Geometry check sheet. Reference: drawing and pictorial views, mm from the part's lowest x, y, z. A direction names the side the tool comes from. Round coordinates to 2 decimals unless told otherwise and drop trailing zeros. Write each loop counter-clockwise with the first axis right and the second up, starting at its lowest first coordinate (ties: lowest second). Pieces come first, ordered by that corner, then holes. Notation, with made-up numbers: M 45.5,32.25 L 74.5,32.25 A22 cw 74.5,55.25 Z; hole C 32.25,-14.5 d3. An arc over 180 degrees is marked long. Put each result on its own line as item: value. Start each with the question number.
(1) Section check A-A on x = 57.5. Record the cut outline in (y, z).
(2) Section check C-C on y = 102.5. Record the cut outline in (x, z), then the cut area to 3 significant figures.
(3) Material ranges on probe 1 along Y at (x, z) = (56, 52.5); probe 2 along Y at (x, z) = (57.5, 54); probe 3 along Z at (x, y) = (7.5, 31.5), recorded low to high.
(4) Tool access check on the marked faces 1 and 2. Record the directions out of +Z, -Z, +X, -X, +Y, -Y that give a thin tool (end or side, any length) a straight path to the whole face; none if there is none.
(5) Mould release check, pull along Y, two halves, no side actions. Record for the marked faces 3, 4 and 5: pulls with the +Y half, pulls with the -Y half, needs draft (parallel to the pull), parting line crosses it, or undercut.
(6) Gauge pin test, flat ends, axial feed: pin 1 (6 mm diameter, centred on x = 102.5, y = 57.5, fed in from +Z); pin 2 (10 mm diameter, centred on x = 22.5, z = 46.5, fed in from +Y); pin 3 (10 mm diameter, centred on x = 62.5, z = 6, fed in from -Y); pin 4 (10 mm diameter, centred on x = 65.5, z = 29, fed in from -Y). Record the tip position at first contact, or that the pin passes through.
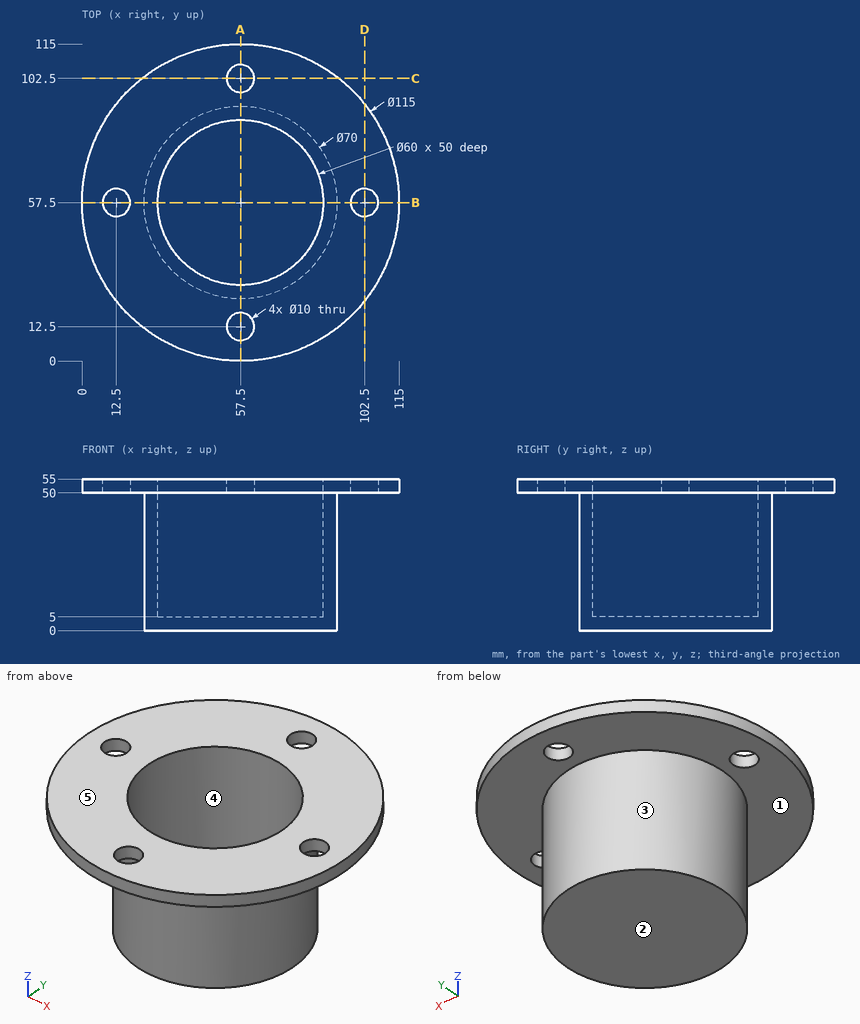
Answers follow:
1. outline: M 0,50 L 7.5,50 L 7.5,55 L 0,55 Z; M 17.5,50 L 22.5,50 L 22.5,0 L 92.5,0 L 92.5,50 L 97.5,50 L 97.5,55 L 87.5,55 L 87.5,5 L 27.5,5 L 27.5,55 L 17.5,55 Z; M 107.5,50 L 115,50 L 115,55 L 107.5,55 Z
2. outline: M 21.71,50 L 52.5,50 L 52.5,55 L 21.71,55 Z; M 62.5,50 L 93.29,50 L 93.29,55 L 62.5,55 Z
2. area: 308 mm^2
3. probe 1: y = 0.02 to 7.73, 17.27 to 27.54, 87.46 to 97.73, 107.27 to 114.98
3. probe 2: y = 0 to 7.5, 17.5 to 27.5, 87.5 to 97.5, 107.5 to 115
3. probe 3: z = 50 to 55
4. face 1: -Z
4. face 2: -Z, +X, -X, +Y, -Y
5. face 3: parting line crosses it
5. face 4: undercut
5. face 5: needs draft
6. pin 1: passes through
6. pin 2: stops at y = 105.65
6. pin 3: stops at y = 22.5
6. pin 4: stops at y = 22.63
